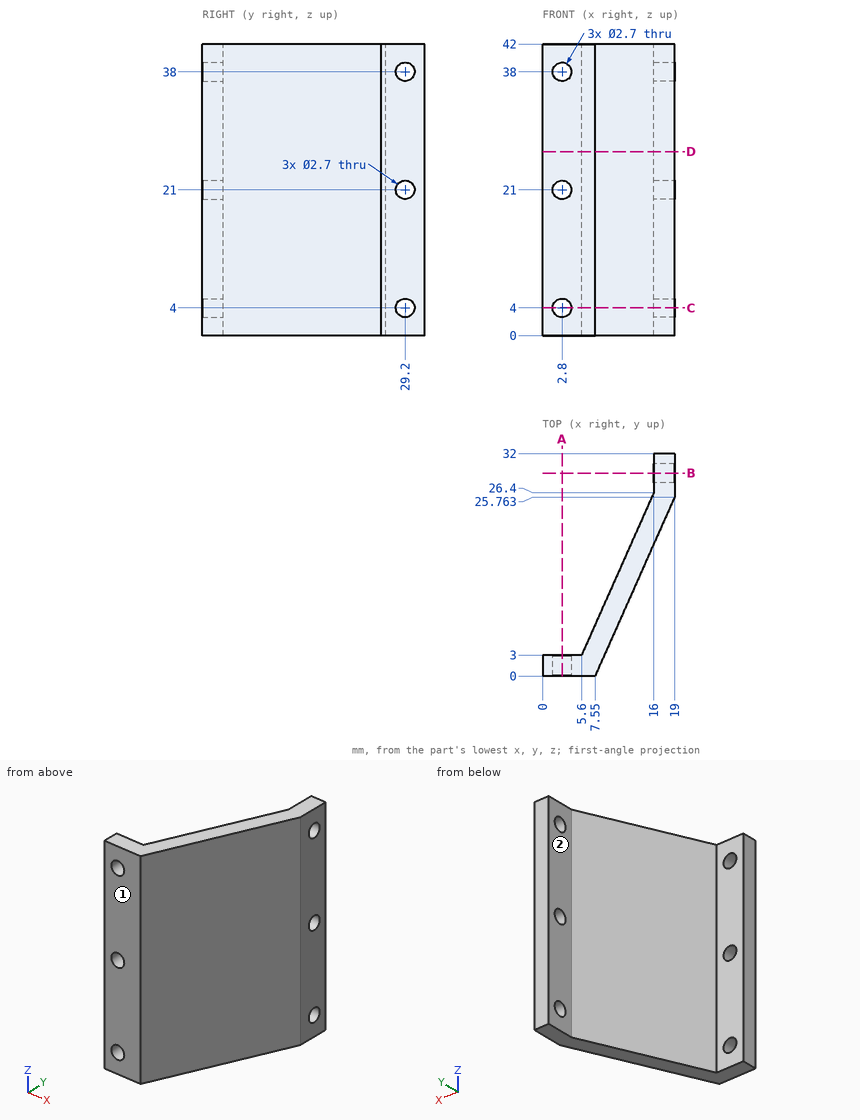
Check sheet for the drawn part. Datum: minimum x, y, z corner. Units: mm. A direction names the side the tool comes from. Give positions to 0.01 mm unless a question says otherwise; leave off trailing zeros. Write each loop counter-clockwise with the first axis right and the second up, starting at its lowest first coordinate (ties: lowest second). Pieces come first, ordered by that corner, then holes. Notation, with made-up numbers: M 40,13.5 L 70,13.5 A26 ccw 70,47.5 Z; hole C 32.25,76.5 d4. An arc over 180 degrees is marked long. Write item = value, one per line.
(1) Access from +Z, -Z, +X, -X, +Y, -Y to the whole of each face (thin tool, end or side, straight path). Record for the marked faces 1 and 2.
Found:
face_1 = +Z, -Z, +X, -X, -Y
face_2 = +Z, -Z, -X, +Y
(2) Sectioned sample at B-B (y = 29.2). Record the cut outline in (x, z), then the cut area to 3 significant figures.
Found:
outline = M 16,0 L 19,0 L 19,2.65 L 16,2.65 Z; M 16,5.35 L 19,5.35 L 19,19.65 L 16,19.65 Z; M 16,22.35 L 19,22.35 L 19,36.65 L 16,36.65 Z; M 16,39.35 L 19,39.35 L 19,42 L 16,42 Z
area = 102 mm2
(3) Material ranges on line 1 (Z direction, x = 2.8, y = 1.15); line 2 (X direction, y = 29.5, z = 8.5); line 3 (X direction, y = 13, z = 33) (1 decimal), recorded low to high.
Found:
line_1 = 0 to 2.65, 5.35 to 19.65, 22.35 to 36.65, 39.35 to 42
line_2 = 16 to 19
line_3 = 10 to 13.3
(4) Sectioned sample at C-C (z = 4). Record the cut outline in (x, y).
Found:
outline = M 0,0 L 1.45,0 L 1.45,3 L 0,3 Z; M 4.15,0 L 7.55,0 L 19,25.76 L 19,27.85 L 16,27.85 L 16,26.4 L 5.6,3 L 4.15,3 Z; M 16,30.55 L 19,30.55 L 19,32 L 16,32 Z
(5) Sectioned sample at D-D (z = 26.5). Record the cut outline in (x, y), then the cut area to 3 significant figures.
Found:
outline = M 0,0 L 7.55,0 L 19,25.76 L 19,32 L 16,32 L 16,26.4 L 5.6,3 L 0,3 Z
area = 118 mm2
(6) Sectioned sample at A-A (x = 2.8). Record the cut outline in (y, z).
Found:
outline = M 0,0 L 3,0 L 3,2.65 L 0,2.65 Z; M 0,5.35 L 3,5.35 L 3,19.65 L 0,19.65 Z; M 0,22.35 L 3,22.35 L 3,36.65 L 0,36.65 Z; M 0,39.35 L 3,39.35 L 3,42 L 0,42 Z
(7) Go/stop test with flat-tipped pins: pin 1 Ø3 at (y, z) = (29.2, 4) entering from -X; pin 2 Ø1.6 at (y, z) = (29.2, 21) entering from +X; pin 3 Ø5 at (y, z) = (22.5, 23.5) entering from +X; pin 4 Ø1 at (y, z) = (25, 32) entering from +X. Record where each tip stops, or that it passes through.
Found:
pin_1 = 16
pin_2 = through
pin_3 = 18.66
pin_4 = 18.88
